The model under review builds one solid part; all positions refer to its coordinate system, in mm. Face numbers are marked on the shaded views. A direction names the side the tool comes from. Coordinates: 2 decimals unless noted, no trailing zeros. Write each loop counter-clockwise with the first axis right and the second up, starting at its lowest first coordinate (ties: lowest second). Pieces come first, ordered by that corner, then holes.
1) For line 1 (X direction, y = 5.25, z = 0); line 2 (X direction, y = 1.5, z = 20.5); line 3 (Z direction, x = 9.5, y = 7.75), list the stretches that pass through material, from the lowest coordinate up.
2) Mouldability with a two-part tool opening along Z and no side actions: class the marked faces 1, 2, 3 and 4 as released by +Z, released by -Z, zero draft, split by the parting line, or undercut.
3) Add section B-B, the plane x = 14. State the section outline as (y, z) points.
4) Machinability: for the marked faces 5 and 6, which of the approach directions +Z, -Z, +X, -X, +Y, -Y give a long, thin tool a straight path to every point of the face, cutting with its end or side? Answer none if there is none.
5) Add section C-C, the plane z = 16. State the section outline as (x, y) points.
6) For P1, Ø6, axis at y = 2.5, z = 19.5, coming from the -X side; P2, Ø1.1, axis at x = 0, y = 3.5, coming from the +Z side; P3, Ø0.7, axis at x = 5, y = 6, coming from the +Z side, all flat-tipped, find the tip position at first contact; note any pin that passes through.
7) Add section D-D, the plane y = 3.75. Give the number of separate pieces and of enclosed holes in the cut face, then the cut area to 3 significant figures.
from build123d import *

# Parameters (mm, degrees)
SKETCH1_R           = 2.5
BOSS_EXTRUDE1_DEPTH = 10
SKETCH2_R           = 2
CUT_EXTRUDE1_DEPTH  = 10
CIRPATTERN1_COUNT   = 3
SKETCH3_R           = 2.5
BOSS_EXTRUDE3_DEPTH = 10


with BuildPart() as part:
    # Sketch1 → Boss-Extrude1 (new body)
    with BuildSketch(Plane(origin=(0, 0, 0), x_dir=(1, 0, 0), z_dir=(0, 1, 0))):
        with BuildLine():
            Line((3.42943918, -9.393558799), (4.197898245, -29.378790113))
            ThreePointArc((4.197898245, -29.378790113), (3.237059632, -30.416474632), (2.199375114, -29.455636019))
            Line((2.199375114, -29.455636019), (1.447231615, -9.894721858))
            ThreePointArc((1.447231615, -9.894721858), (0.350023332, -9.993872306), (-0.751433173, -9.971727442))
            Line((-0.751433173, -9.971727442), (0.000999669, -29.540166516))
            ThreePointArc((0.000999669, -29.540166516), (-0.935779597, -30.318112399), (-1.929530696, -29.614398009))
            Line((-1.929530696, -29.614398009), (-2.697989761, -9.629166695))
            ThreePointArc((-2.697989761, -9.629166695), (-8.461744243, -5.329060364), (-9.849780142, 1.726797949))
            Line((-9.849780142, 1.726797949), (-27.541727692, 11.053908534))
            ThreePointArc((-27.541727692, 11.053908534), (-27.959969541, 12.404861441), (-26.609016634, 12.823103289))
            Line((-26.609016634, 12.823103289), (-9.2926963, 3.694021585))
            ThreePointArc((-9.2926963, 3.694021585), (-8.829958965, 4.693807055), (-8.260052699, 5.636623938))
            Line((-8.260052699, 5.636623938), (-25.58303447, 14.769217519))
            ThreePointArc((-25.58303447, 14.769217519), (-25.788365734, 15.969465103), (-24.682055646, 16.478221605))
            Line((-24.682055646, 16.478221605), (-6.990108095, 7.15111102))
            ThreePointArc((-6.990108095, 7.15111102), (-0.384229532, 9.992615657), (6.420340962, 7.66676085))
            Line((6.420340962, 7.66676085), (23.343829448, 18.324881579))
            ThreePointArc((23.343829448, 18.324881579), (24.722909908, 18.011613191), (24.40964152, 16.63253273))
            Line((24.40964152, 16.63253273), (7.845464685, 6.200700273))
            ThreePointArc((7.845464685, 6.200700273), (8.479935633, 5.300065251), (9.011485871, 4.335103505))
            Line((9.011485871, 4.335103505), (25.582034801, 14.770948997))
            ThreePointArc((25.582034801, 14.770948997), (26.724145331, 14.348647296), (26.611586342, 13.136176404))
            Line((26.611586342, 13.136176404), (9.688097856, 2.478055676))
            ThreePointArc((9.688097856, 2.478055676), (8.845973775, -4.663555293), (3.42943918, -9.393558799))
        make_face()
        Circle(SKETCH1_R, mode=Mode.SUBTRACT)
    extrude(amount=BOSS_EXTRUDE1_DEPTH)

    # Sketch2 → Cut-Extrude1 (cut)
    with BuildSketch(Plane(origin=(3.063714471, 0, -0.117803948), x_dir=(-0.038422953, 0, -0.999261566), z_dir=(0.999261566, 0, -0.038422953))):
        with Locations((-24.518391454, 5)):
            Circle(SKETCH2_R)
    cut_extrude1 = extrude(amount=-CUT_EXTRUDE1_DEPTH, mode=Mode.SUBTRACT)

    # CirPattern1: Cut-Extrude1 ×3 about axis
    cirpattern1_axis = Axis((0, 10, 0), (0, -1, 0))
    for i in range(1, CIRPATTERN1_COUNT):
        add(cut_extrude1.rotate(cirpattern1_axis, i * 360 / CIRPATTERN1_COUNT), mode=Mode.SUBTRACT)

    # Sketch3 → Boss-Extrude3 (add)
    with BuildSketch(Plane(origin=(0, 10, 0), x_dir=(1, 0, 0), z_dir=(0, 1, 0))):
        Polygon((11.5901527, 0), (5.79507635, 10.037366672), (-5.79507635, 10.037366672), (-11.5901527, 0), (-5.79507635, -10.037366672), (5.79507635, -10.037366672), align=None)
        Circle(SKETCH3_R, mode=Mode.SUBTRACT)
    extrude(amount=-BOSS_EXTRUDE3_DEPTH)


solid = part.part
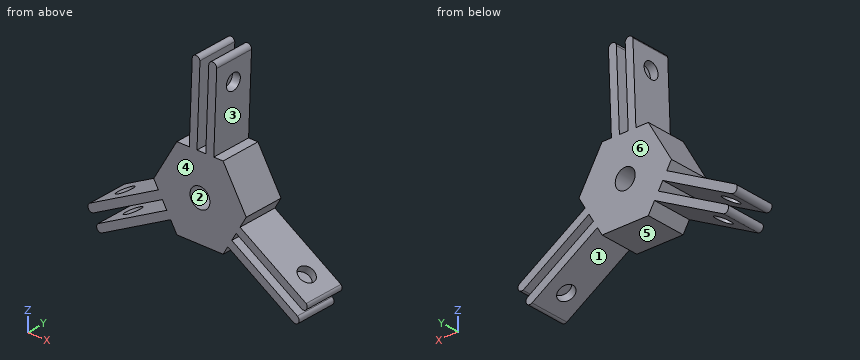
Geometry results:
1. line 1: x = -11.59 to -2.5, 2.5 to 11.59
1. line 2: x = -2.28 to -0.35, 1.86 to 3.86
1. line 3: z = -9.61 to -7.24, -4.64 to 3.62
2. face 1: released by -Z
2. face 2: undercut
2. face 3: undercut
2. face 4: zero draft
3. outline: (0, -12.44) - (10, -12.44) - (10, -10.08) - (0, -10.08) - close; (0, -7.48) - (10, -7.48) - (10, -5.19) - (0, -5.19) - close
4. face 5: -Z, +Y, -Y
4. face 6: +Z, -Z, +X, -X, +Y
5. outline: (-2.45, 0) - (-0.52, 0) - (-0.52, 10) - (-2.45, 10) - close; (1.68, 0) - (3.68, 0) - (3.68, 10) - (1.68, 10) - close
6. P1: stops at x = -2.43
6. P2: stops at z = 30.22
6. P3: stops at z = 10.04
7. separate pieces: 7
7. enclosed holes: 1
7. area: 530 mm2
